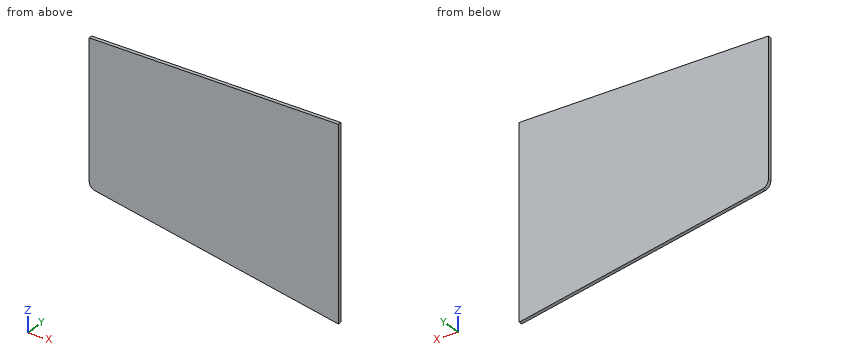
```python
from build123d import *

# Parameters (mm, degrees)
BOSS_EXTRUDE1_DEPTH = 6.35


with BuildPart() as part:
    # Sketch1 → Boss-Extrude1 (new body)
    with BuildSketch(Plane(origin=(0, 0, 0), x_dir=(1, 0, 0), z_dir=(0, 1, 0))):
        with BuildLine():
            Line((0, 0), (437.02224, 0))
            Line((437.02224, 0), (437.02224, 335.28))
            Line((437.02224, 335.28), (10.307768658, 253.437009611))
            ThreePointArc((10.307768658, 253.437009611), (2.910430601, 249.054735438), (0, 240.964350344))
            Line((0, 240.964350344), (0, 0))
        make_face()
    extrude(amount=BOSS_EXTRUDE1_DEPTH)


solid = part.part
```
For this review, take the finished solid that the model builds, in its own axes (mm). Coordinates: 2 decimals unless noted, no trailing zeros. Write each loop counter-clockwise with the first axis right and the second up, starting at its lowest first coordinate (ties: lowest second). Pieces come first, ordered by that corner, then holes. Notation, with made-up numbers: (67.25, -18) - (116.25, -18) arc R21 ccw to (116.25, 4) - close; hole circle Ø2 at (18, 62). An arc over 180 degrees is marked (long way). Answer in a Markdown table with one row per item. Add a question column.
Q1. We need section C-C, the plane z = -274. State the section outline as (x, y) points, and give its area (3 significant figures).
Q2. For probe 1 along Z at (x, y) = (277, 5.75); probe 2 along Z at (x, y) = (357, 1), list the stretches that pass through material, from the lowest coordinate up.
Q3. We need section B-B, the plane x = 215. State the section outline as (y, z) points.
Q4. We need section A-A, the plane y = 3.5. State the section outline as (x, z) points, and give its area (3 significant figures).
Answer list:
| question | item | result |
|---|---|---|
| 1 | outline | (117.52, 0) - (437.02, 0) - (437.02, 6.35) - (117.52, 6.35) - close |
| 1 | area | 2,030 mm2 |
| 2 | probe 1 | z = -304.59 to 0 |
| 2 | probe 2 | z = -319.93 to 0 |
| 3 | outline | (0, -292.7) - (6.35, -292.7) - (6.35, 0) - (0, 0) - close |
| 4 | outline | (0, -240.96) arc R12.7 ccw to (10.31, -253.44) - (437.02, -335.28) - (437.02, 0) - (0, 0) - close |
| 4 | area | 128,000 mm2 |
